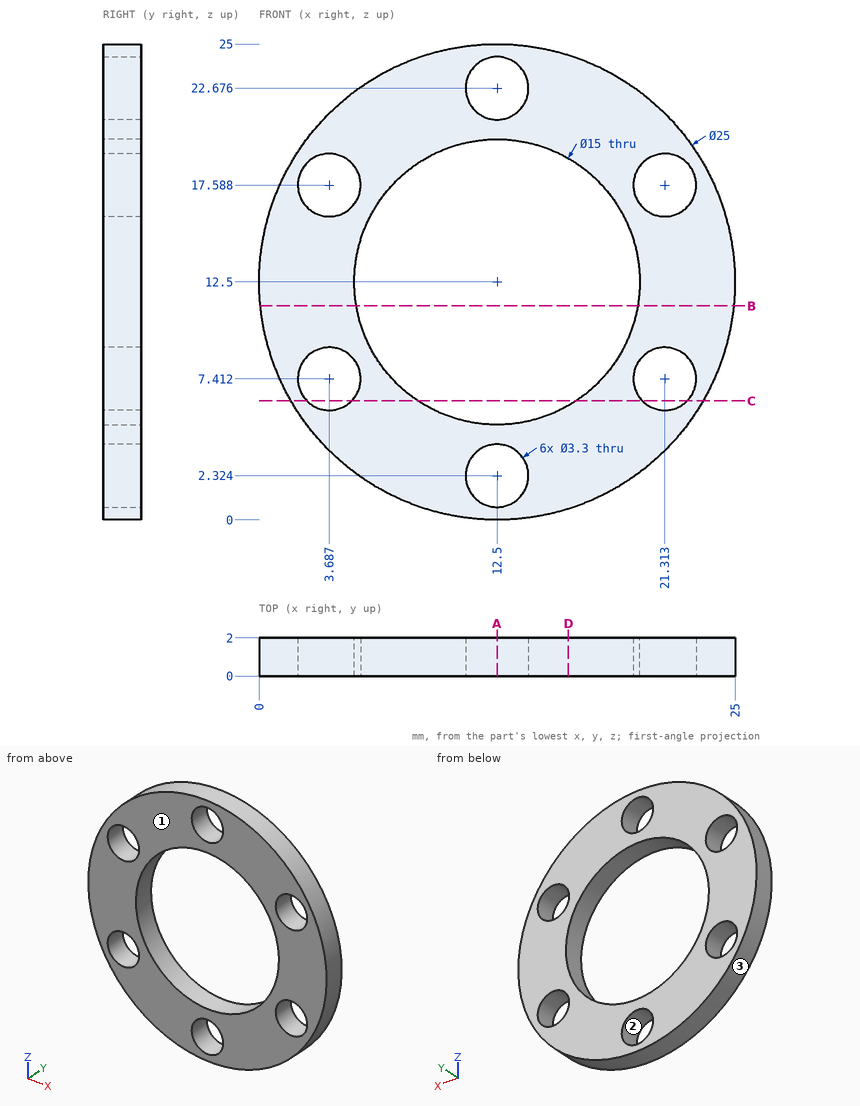
Here's the drawing with two shaded views (mm, measured from the low corner). I have some questions. Give positions to 0.01 mm unless a question says otherwise; leave off trailing zeros. Loops run counter-clockwise (first coordinate to the right, second up) from the corner with the lowest first, then second, coordinate; pieces in that order, holes last. Notation, with made-up numbers: (-18.75, 7) -> (37.25, 7) arc R26 cw to (37.25, 24) -> close; hole circle Ø9 at (4, -25). An arc over 180 degrees is marked (long way). One line per item, written item: value.
Q1. Suppose I cut it at D-D on x = 16.25. Please give me the cut outline in (y, z) (1 decimal).
Answers follow:
outline: (0, 0.6) -> (2, 0.6) -> (2, 6) -> (0, 6) -> close; (0, 19) -> (2, 19) -> (2, 24.4) -> (0, 24.4) -> close
Q2. Suppose I cut it at B-B on z = 11.25. Please give me the cut outline in (x, y) (1 decimal).
Answers follow:
outline: (0.1, 0) -> (5.1, 0) -> (5.1, 2) -> (0.1, 2) -> close; (19.9, 0) -> (24.9, 0) -> (24.9, 2) -> (19.9, 2) -> close
Q3. Suppose I cut it at A-A on x = 12.5. Please give me the cut outline in (y, z).
Answers follow:
outline: (0, 0) -> (2, 0) -> (2, 0.67) -> (0, 0.67) -> close; (0, 3.97) -> (2, 3.97) -> (2, 5) -> (0, 5) -> close; (0, 20) -> (2, 20) -> (2, 21.03) -> (0, 21.03) -> close; (0, 24.33) -> (2, 24.33) -> (2, 25) -> (0, 25) -> close
Q4. If I drill on line 1 along Z through (x, y) = (21, 0.25) (1 decimal); line 2 along X through (y, z) = (1.8, 6.25) (1 decimal); line 3 along Z through (x, y) = (11.25, 0.7) (1 decimal), over which ranges is the centre line in solid material (lowest first)?
Answers follow:
line 1: 3.3 to 5.8, 9 to 16, 19.2 to 21.7
line 2: 1.7 to 2.5, 4.9 to 8.4, 16.6 to 20.1, 22.5 to 23.3
line 3: 0.1 to 1.2, 3.4 to 5.1, 19.9 to 21.6, 23.8 to 24.9
Q5. I'm going to push a flat-ended pin straight in: pin 1 Ø3 at (x, z) = (21.31, 17.59) entering from -Y. Where does the tip first touch, or does it pass through?
Answers follow:
pin 1: through
Q6. Suppose I cut it at C-C on z = 6.25. Please give me the cut outline in (x, y) (1 decimal).
Answers follow:
outline: (1.7, 0) -> (2.5, 0) -> (2.5, 2) -> (1.7, 2) -> close; (4.9, 0) -> (8.4, 0) -> (8.4, 2) -> (4.9, 2) -> close; (16.6, 0) -> (20.1, 0) -> (20.1, 2) -> (16.6, 2) -> close; (22.5, 0) -> (23.3, 0) -> (23.3, 2) -> (22.5, 2) -> close
Q7. We'd pull the mould along X, two halves only. Please class the marked faces 1, 2 and 3: pulls with the +X half, pulls with the -X half, needs draft (parallel to the pull), parting line crosses it, or undercut.
Answers follow:
face 1: needs draft
face 2: undercut
face 3: parting line crosses it
